Can you work these out from the drawing? Everything is in mm from the part's minimum corner. Coordinates: 2 decimals unless noted, no trailing zeros. Order: outer loops, then holes, each group sorted by start corner. A loop starts at its lowest first (then second) coordinate and runs counter-clockwise, first axis right, second up. Notation, with made-up numbers: (50, 26.5) - (90, 26.5) arc R21 cw to (90, 54.5) - close; hole circle Ø8 at (-21, 29.25). An arc over 180 degrees is marked (long way). One line per item, written item: value.
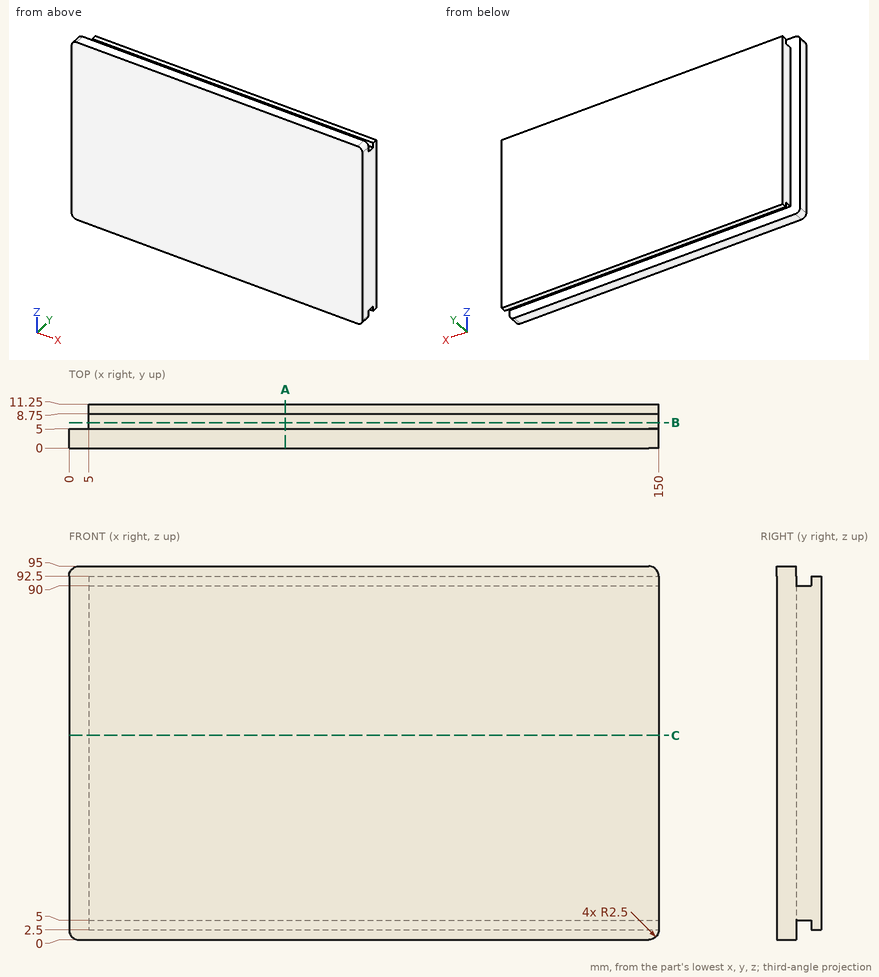
Item 1: I want a section at A-A on x = 55. Please give me the cut outline in (y, z).
Conclusion:
outline: (0, 0) - (5, 0) - (5, 5) - (8.75, 5) - (8.75, 2.5) - (11.25, 2.5) - (11.25, 92.5) - (8.75, 92.5) - (8.75, 90) - (5, 90) - (5, 95) - (0, 95) - close
Item 2: I want a section at B-B on y = 6.5. Please give me the cut outline in (x, z), then the cut area to 3 significant figures.
Conclusion:
outline: (5, 5) - (150, 5) - (150, 90) - (5, 90) - close
area: 12,300 mm²
Item 3: If I drill on probe 1 along Y at (x, z) = (135, 4); probe 2 along X at (y, z) = (10, 22); probe 3 along Z at (x, y) = (77.5, 7.25), over which ranges is the centre line in solid material (lowest first)?
Conclusion:
probe 1: 0 to 5, 8.75 to 11.25
probe 2: 5 to 150
probe 3: 5 to 90
Item 4: I'm going to push flat-ended pins straight in: pin 1 Ø1.9 at (y, z) = (9.5, 29.5) entering from -X; pin 2 Ø1 at (x, y) = (60.5, 6.5) entering from -Z; pin 3 Ø3 at (x, y) = (109, 10) entering from +Z. Where does each tip first touch, or does it pass through?
Conclusion:
pin 1: x = 5
pin 2: z = 5
pin 3: z = 92.5
Item 5: I want a section at C-C on z = 52. Please give me the cut outline in (x, y), then the cut area to 3 significant figures.
Conclusion:
outline: (0, 0) - (150, 0) - (150, 11.25) - (5, 11.25) - (5, 5) - (0, 5) - close
area: 1,660 mm²
